```python
from build123d import *

# Parameters (mm, degrees)
F0_R         = 8
F1_DEPTH     = 3.7
F2_R         = 6
F3_DEPTH     = 6
F4_R         = 8
F5_DEPTH     = 3
F6_W         = 4
F6_H         = 1.5
F8_R         = 2.1
F9_DEPTH     = 42.7
F10_R        = 4
F11_DEPTH    = 6
F12_S5_R     = 4
F12_T6_DEPTH = 7
F13_R        = 3
F14_DEPTH    = 14.8
F15_S5_R     = 3
F15_T6_DEPTH = 6


# Not quite as in the source:
# - a fillet or chamfer that OpenCascade refuses, or shapes differently, is made with other operations: its cross-section is extruded or revolved along the edge and cut away or added


with BuildPart() as f1:
    # F0 (on Top) → F1 (new body)
    with BuildSketch(Plane.XY):
        Circle(F0_R)
    extrude(amount=-F1_DEPTH)

    # F2 (on face) → F3 (join)
    with BuildSketch(Plane(origin=(0, 0, -3.7), x_dir=(1, 0, 0), z_dir=(0, 0, -1))):
        Circle(F2_R)
    extrude(amount=F3_DEPTH)

    # F4 (on face) → F5 (join)
    with BuildSketch(Plane(origin=(0, 0, -9.7), x_dir=(1, 0, 0), z_dir=(0, 0, -1))):
        Circle(F4_R)
    extrude(amount=F5_DEPTH)

    # F6 (on Front) → F7 (revolve)
    with BuildSketch(Plane.XZ):
        with Locations((2, -13.45)):
            Rectangle(F6_W, F6_H)
        Polygon((4, -14.2), (0, -14.2), (0, -15.2), (4.0727272727, -15.2), (8, -15.2), (8, -14.2), align=None)
        Polygon((4.0727272727, -15.2), (0, -15.2), (0, -16.7), (4.1818181818, -16.7), align=None)
        Polygon((4.1818181818, -16.7), (0, -16.7), (0, -17.7), (4.2545454545, -17.7), (11.15, -17.7), (11.15, -16.7), align=None)
        Polygon((4.2545454545, -17.7), (0, -17.7), (0, -19.2), (4.3636363636, -19.2), align=None)
        Polygon((4.3636363636, -19.2), (0, -19.2), (0, -20.2), (4.4363636364, -20.2), (11.15, -20.2), (11.15, -19.2), align=None)
        Polygon((4.4363636364, -20.2), (0, -20.2), (0, -21.7), (4.5454545455, -21.7), align=None)
        Polygon((4.5454545455, -21.7), (0, -21.7), (0, -22.7), (4.6181818182, -22.7), (11.15, -22.7), (11.15, -21.7), align=None)
        Polygon((4.6181818182, -22.7), (0, -22.7), (0, -24.2), (4.7272727273, -24.2), align=None)
        Polygon((4.7272727273, -24.2), (0, -24.2), (0, -25.2), (4.8, -25.2), (11.15, -25.2), (11.15, -24.2), align=None)
        Polygon((4.8, -25.2), (0, -25.2), (0, -26.7), (4.9090909091, -26.7), align=None)
        Polygon((4.9090909091, -26.7), (0, -26.7), (0, -27.7), (4.9818181818, -27.7), (11.15, -27.7), (11.15, -26.7), align=None)
        Polygon((4.9818181818, -27.7), (0, -27.7), (0, -29.2), (5.0909090909, -29.2), align=None)
        Polygon((5.0909090909, -29.2), (0, -29.2), (0, -30.2), (5.1636363636, -30.2), (11.15, -30.2), (11.15, -29.2), align=None)
        Polygon((5.1636363636, -30.2), (0, -30.2), (0, -31.7), (5.2727272727, -31.7), align=None)
        Polygon((5.2727272727, -31.7), (0, -31.7), (0, -32.7), (5.3454545455, -32.7), (11.15, -32.7), (11.15, -31.7), align=None)
        Polygon((5.3454545455, -32.7), (0, -32.7), (0, -34.2), (5.4545454545, -34.2), align=None)
        Polygon((5.4545454545, -34.2), (0, -34.2), (0, -35.2), (5.5272727273, -35.2), (11.15, -35.2), (11.15, -34.2), align=None)
        Polygon((5.5272727273, -35.2), (0, -35.2), (0, -36.7), (5.6363636364, -36.7), align=None)
        Polygon((5.6363636364, -36.7), (0, -36.7), (0, -37.7), (5.7090909091, -37.7), (11.15, -37.7), (11.15, -36.7), align=None)
        Polygon((5.7090909091, -37.7), (0, -37.7), (0, -39.2), (5.8181818182, -39.2), align=None)
        Polygon((5.8181818182, -39.2), (0, -39.2), (0, -40.2), (5.8909090909, -40.2), (11.15, -40.2), (11.15, -39.2), align=None)
        Polygon((5.8909090909, -40.2), (0, -40.2), (0, -41.7), (6, -41.7), align=None)
        Polygon((6, -41.7), (0, -41.7), (0, -42.7), (11.15, -42.7), (11.15, -41.7), align=None)
    revolve(axis=Axis((0, 0, -6.35), (0, 0, -1)))

    # F8 (on face) → F9 (cut)
    with BuildSketch(Plane.XY):
        Circle(F8_R)
    extrude(amount=-F9_DEPTH, mode=Mode.SUBTRACT)

    # F10 (on face) → F11 (cut)
    with BuildSketch(Plane.XY):
        Circle(F10_R)
    extrude(amount=-F11_DEPTH, mode=Mode.SUBTRACT)

    # F12: chamfer of 2 on 1 edges, made by hand


with BuildPart() as f12_tool2:
    # F12_s3 → F12_t4 (revolve)
    with BuildSketch(Plane.XZ):
        Polygon((4.1, -6), (2.1, -8), (2.1, -6), align=None)
    revolve(axis=Axis((0, 0, -6), (0, 0, 1)))

    # F12_s5 → F12_t6 (intersect, symmetric)
    with BuildSketch(Plane.XY.offset(-7)):
        Circle(F12_S5_R)
    extrude(amount=F12_T6_DEPTH, both=True, mode=Mode.INTERSECT)


with BuildPart() as f1_1:
    add(f1.part)

    # F12_t1: cut F12_tool2
    add(f12_tool2.part, mode=Mode.SUBTRACT)

    # F13 (on face) → F14 (cut)
    with BuildSketch(Plane(origin=(0, 0, -42.7), x_dir=(1, 0, 0), z_dir=(0, 0, -1))):
        Circle(F13_R)
    extrude(amount=-F14_DEPTH, mode=Mode.SUBTRACT)

    # F15: chamfer of 1 on 1 edges, made by hand


with BuildPart() as f15_tool2:
    # F15_s3 → F15_t4 (revolve)
    with BuildSketch(Plane.XZ):
        Polygon((2.1, -26.9), (3.1, -27.9), (2.1, -27.9), align=None)
    revolve(axis=Axis((0, 0, -27.9), (0, 0, 1)))

    # F15_s5 → F15_t6 (intersect, symmetric)
    with BuildSketch(Plane.XY.offset(-27.4)):
        Circle(F15_S5_R)
    extrude(amount=F15_T6_DEPTH, both=True, mode=Mode.INTERSECT)


with BuildPart() as f1_2:
    add(f1_1.part)

    # F15_t1: cut F15_tool2
    add(f15_tool2.part, mode=Mode.SUBTRACT)


solid = f1_2.part
```
Here's how the part is built. I have some questions about the finished solid (model axes, mm). A direction names the side the tool comes from. Give positions to 0.01 mm unless a question says otherwise; leave off trailing zeros. Loops run counter-clockwise (first coordinate to the right, second up) from the corner with the lowest first, then second, coordinate; pieces in that order, holes last. Notation, with made-up numbers: M 54,20 L 112,20 A27 cw 112,44 Z; hole C -14.75,5.25 d10. An arc over 180 degrees is marked long. Put each result on its own line as item: value. Start each with the question number.
(1) Will these pins go through, and if not, where does the flat tip stop? pin 1 Ø1 at (y, z) = (-8, -35.5) entering from +X; pin 2 Ø5 at (x, y) = (1, -0.5) entering from -Z; pin 3 Ø6 at (x, z) = (3.5, -17) entering from -Y; pin 4 Ø3.5 at (x, y) = (0, 0) entering from -Z.
(2) For faces 4 (the cylindrical face through (10.635, -3.349, -39.693)), 5 (the cylindrical face through (-1.73, 7.81, -11.18)), 6 (the cylindrical face through (-0.65, -2.93, -35.15)), 7 (the flat face through (-2, 6, -3.7)), which set-ups out of +Z, -Z, +X, -X, +Y, -Y let a thin tool reach every point of the face, with its end or its side?
(3) I need wall thicknesses on line 1 along Y through (x, z) = (0, -12.25); line 2 along X through (y, z) = (0, -40); line 3 along Y through (x, z) = (0, -2.75). Which ranges of each line are inside material? Lowest first, please. Write a range as [from, to].
(4) If we mould it in two halves opening along Z, with no side actions, what happens to faces 1 (the cylindrical face through (10.635, -3.349, -34.693)), 2 (the flat face through (-2, -6, -9.7)), 3 (the conical face through (-0.53, -4.07, -15.61))? For each: +Z half, -Z half, draft (parallel to the pull), parting line (faces both ways), or undercut.
(5) I want a section at B-B on y = 10.25. State how many separate pieces and enclosed holes the cut face has, then the cut area to 3 significant figures.
(6) I want a section at A-A on z = -7. Please give me the cut outline in (x, y), then the cut area to 3 significant figures.
Answer block:
1. pin 1: x = 8.16
1. pin 2: z = -42.7
1. pin 3: y = -11.14
1. pin 4: through
2. face 4: +Z, -Z
2. face 5: +Z
2. face 6: -Z
2. face 7: none
3. line 1: [-8, -2.1], [2.1, 8]
3. line 2: [-11.15, -3], [3, 11.15]
3. line 3: [-8, -4], [4, 8]
4. face 1: draft
4. face 2: undercut
4. face 3: undercut
5. separate pieces: 11
5. enclosed holes: 0
5. area: 96.5 mm^2
6. outline: C 0,0 d12; hole C 0,0 d6.2
6. area: 82.9 mm^2
